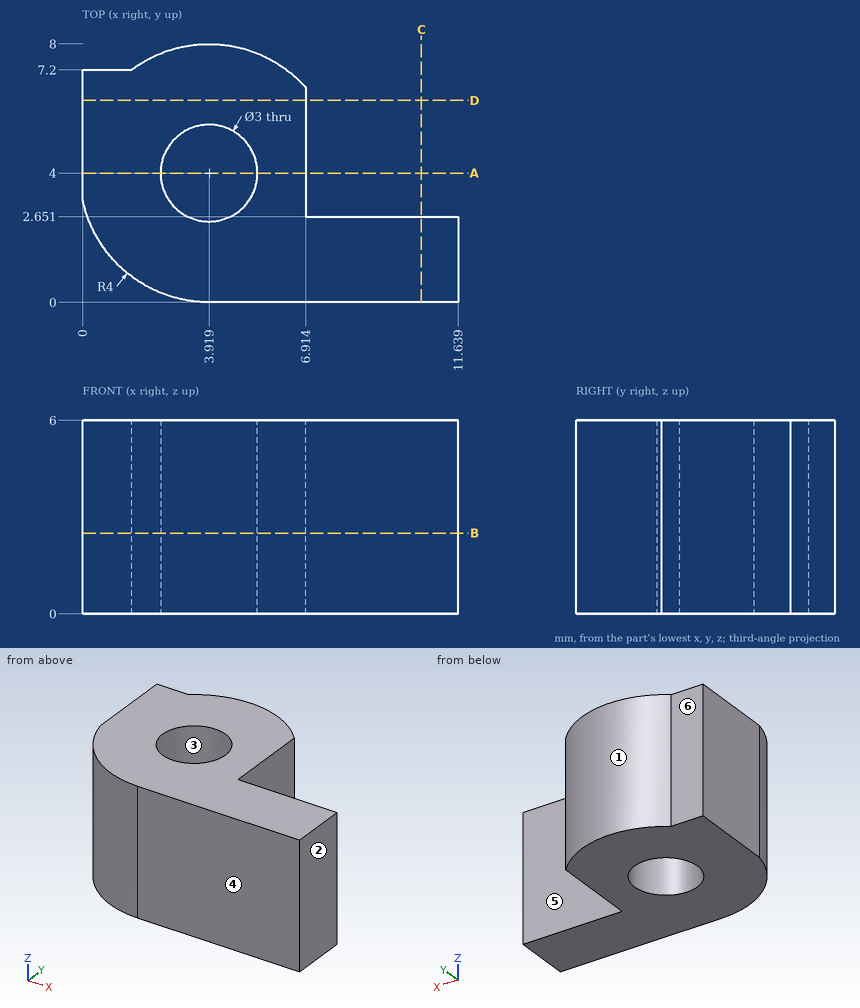
Source: three-view drawing plus pictorial views. Frame: mm from the lowest corner of the part. A direction names the side the tool comes from. Give positions to 0.01 mm unless a question says otherwise; leave off trailing zeros. Order: outer loops, then holes, each group sorted by start corner. A loop starts at its lowest first (then second) coordinate and runs counter-clockwise, first axis right, second up. Notation, with made-up numbers: (-16, 7.5) - (36, 7.5) arc R26 ccw to (36, 22.5) - close; hole circle Ø8 at (47, 19). An arc over 180 degrees is marked (long way). Put each result on its own line as item: value.
Item 1: Ray query, L1, parallel to Y at x = 4, z = 2.9; L2, parallel to X at y = 6.25, z = 3.7 (1 decimal); L3, parallel to Y at x = 9.75, z = 4.3. Return the intervals inside material, ascending. Write a range as from..to.
Found:
L1: y = 0..2.5, 5.5..8
L2: x = 0..6.9
L3: y = 0..2.65
Item 2: Section query B-B, the plane z = 2.5. Return loops of the section in (x, y) (1 decimal).
Found:
outline: (0, 3.2) arc R4 ccw to (3.9, 0) - (11.6, 0) - (11.6, 2.7) - (6.9, 2.7) - (6.9, 6.7) arc R4 ccw to (1.5, 7.2) - (0, 7.2) - close; hole circle Ø3 at (3.9, 4)
Item 3: Section query A-A, the plane y = 4. Return loops of the section in (x, z) (1 decimal).
Found:
outline: (0, 0) - (2.4, 0) - (2.4, 6) - (0, 6) - close; (5.4, 0) - (6.9, 0) - (6.9, 6) - (5.4, 6) - close
Item 4: Contact query for flat-ended pins moving along their axis: pin 1 (1.2 mm diameter, centred on y = 5, z = 2.5, fed in from +X); pin 2 (2 mm diameter, centred on x = 8, z = 4, fed in from +Y); pin 3 (2.5 mm diameter, centred on x = 3.92, y = 4, fed in from -Z); pin 4 (1.7 mm diameter, centred on x = 0.5, z = 2, fed in from +Y). Output: stop coordinate, or through.
Found:
pin 1: stops at x = 6.91
pin 2: stops at y = 2.65
pin 3: passes through
pin 4: stops at y = 7.2
Item 5: Access query for the marked faces 4, 5 and 6. Directions: +Z, -Z, +X, -X, +Y, -Y. A direction counts if a zero-diameter tool reaches every point of the face in a straight line with its end or side. Return the directions, or none.
Found:
face 4: +Z, -Z, +X, -X, -Y
face 5: +Z, -Z, +X, +Y
face 6: +Z, -Z, -X, +Y
Item 6: Draft query along Y for the marked faces 1, 2 and 3. Return one class per face: +Y half, -Y half, draft (parallel to the pull), parting line (faces both ways), or undercut.
Found:
face 1: +Y half
face 2: draft
face 3: undercut
Item 7: Section query C-C, the plane x = 10.5. Return loops of the section in (y, z), then the cut area to 3 significant figures.
Found:
outline: (0, 0) - (2.65, 0) - (2.65, 6) - (0, 6) - close
area: 15.9 mm^2
Item 8: Section query D-D, the plane y = 6.25. Return loops of the section in (x, z) (1 decimal).
Found:
outline: (0, 0) - (6.9, 0) - (6.9, 6) - (0, 6) - close
